Part model, mm, in its own coordinate system. A direction names the side the tool comes from. Give positions to 0.01 mm unless a question says otherwise; leave off trailing zeros. Order: outer loops, then holes, each group sorted by start corner. A loop starts at its lowest first (then second) coordinate and runs counter-clockwise, first axis right, second up.
1. Mould opens along X. For faces 3 (the conical face through (-188.425, -33.482, 80.181)), 4 (the flat face through (-2, -281.94, 2)), 5 (the conical face through (-55.172, -4.131, -248.455)) say: +X half, -X half, draft (parallel to the pull), parting line (faces both ways), or undercut.
2. Probe line 1 (X direction, y = -30.5, z = 107); line 2 (Y direction, x = 43.5, z = 144); line 3 (X direction, y = -26.5, z = 193). List the from-to ranges inside material, lowest first.
3. Slice it at C-C on z = 116. Give the number of separate pieces and of enclosed holes in the cut face, and give its area (3 significant figures).
4. Drop flat-ended pins along their axis: pin 1 Ø8 at (x, z) = (170.5, 156.5) entering from -Y; pin 2 Ø5 at (y, z) = (-108.5, -61) entering from -X; pin 3 Ø6 at (x, y) = (32, -121.5) entering from +Z. Give the stop position or say it passes through.
5. Slice it at B-B on y = -22. List the corners of the cut face in (x, z), and give its area (3 significant figures).
6. Slice it at D-D on y = -148.5. List the corners of the cut face in (x, z).
7. Slice it at A-A on x = 0. List the corners of the cut face in (y, z).
8. Which spindle directions (+Z, -Z, +X, -X, +Y, -Y) get a long thin tool onto all of the face, cutting with end or side? Do faces 1 (the flat face through (113, -66.04, -113)), 2 (the conical face through (-155.319, -33.482, -119.635)). Say none if no direction does.
from build123d import *

# Parameters (mm, degrees)
F0_R     = 254
F0_R_2   = 30.0836769803
F1_DEPTH = 66.04
F1_TAPER = -7
F2_R     = 142.8310706252
F3_DEPTH = 215.9


with BuildPart() as f1:
    # F0 (on Front) → F1 (new body)
    with BuildSketch(Plane.XZ):
        Circle(F0_R)
        with Locations((-169.2818999115, -97.7349504828)):
            Circle(F0_R_2, mode=Mode.SUBTRACT)
        with Locations((0, -195.4699009657)):
            Circle(F0_R_2, mode=Mode.SUBTRACT)
        with Locations((169.2818999115, -97.7349504828)):
            Circle(F0_R_2, mode=Mode.SUBTRACT)
        with Locations((-169.2818999115, 97.7349504828)):
            Circle(F0_R_2, mode=Mode.SUBTRACT)
        with Locations((169.2818999115, 97.7349504828)):
            Circle(F0_R_2, mode=Mode.SUBTRACT)
        with Locations((0, 195.4699009657)):
            Circle(F0_R_2, mode=Mode.SUBTRACT)
    extrude(amount=F1_DEPTH, taper=F1_TAPER)

    # F2 (on face) → F3 (join)
    with BuildSketch(Plane.XZ.offset(66.04)):
        Circle(F2_R)
    extrude(amount=F3_DEPTH)


solid = f1.part
Data:
1. face 3: undercut
1. face 4: draft
1. face 5: parting line
2. line 1: x = -234.49 to -193.94, -144.63 to 144.63, 193.94 to 234.49
2. line 2: y = -66.04 to 0
2. line 3: x = -170.09 to -26.72, 26.72 to 170.09
3. separate pieces: 3
3. enclosed holes: 0
3. area: 61,600 mm2
4. pin 1: stops at y = -66.04
4. pin 2: stops at x = -130.3
4. pin 3: stops at z = 139.86
5. outline: circle Ø513.4 at (0, 0); hole circle Ø54.76 at (-169.28, -97.73); hole circle Ø54.76 at (-169.28, 97.73); hole circle Ø54.76 at (0, -195.47); hole circle Ø54.76 at (0, 195.47); hole circle Ø54.76 at (169.28, -97.73); hole circle Ø54.76 at (169.28, 97.73)
5. area: 193,000 mm2
6. outline: circle Ø285.66 at (0, 0)
7. outline: (-281.94, -142.83) - (-66.04, -142.83) - (-66.04, -173.49) - (0, -165.39) - (0, 165.39) - (-66.04, 173.49) - (-66.04, 142.83) - (-281.94, 142.83) - close; (-66.04, -262.11) - (0, -254) - (0, -225.55) - (-66.04, -217.44) - close; (-66.04, 217.44) - (0, 225.55) - (0, 254) - (-66.04, 262.11) - close
8. face 1: -Y
8. face 2: +Y
